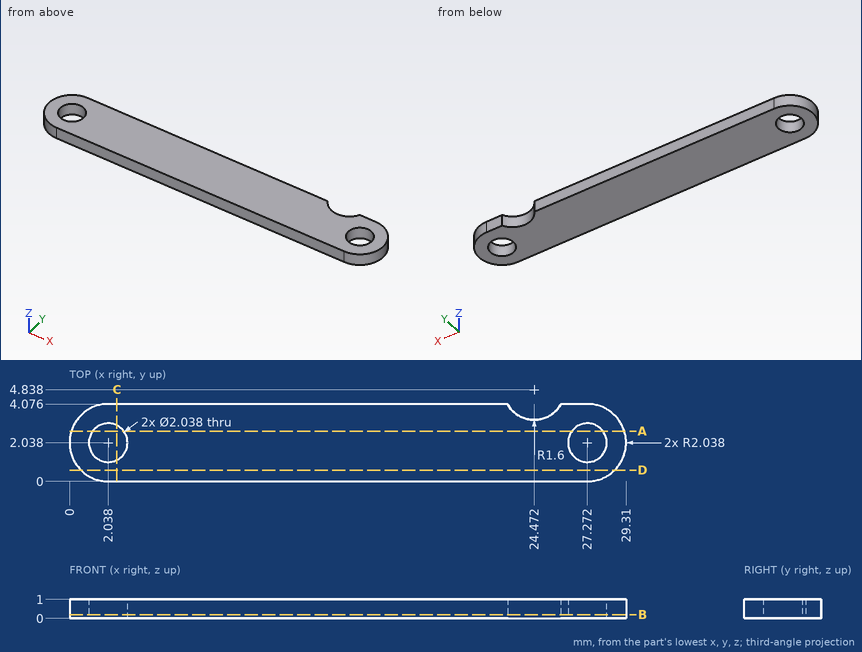
Check sheet for the drawn part. Datum: minimum x, y, z corner. Units: mm. Round coordinates to 2 decimals unless told otherwise and drop trailing zeros. Order: outer loops, then holes, each group sorted by start corner. A loop starts at its lowest first (then second) coordinate and runs counter-clockwise, first axis right, second up. Notation, with made-up numbers: M 20.5,-33.75 L 24.5,-33.75 A21 ccw 24.5,0.25 Z; hole C -32.75,74 d2. An arc over 180 degrees is marked long. Write each question's results on one line, items separated by ' | '. Start each with the question number.
1. Cross-section at D-D on y = 0.6. Record the boundary of the cut face in (x, z).
2. Cross-section at A-A on y = 2.65. Record the boundary of the cut face in (x, z).
3. Cross-section at B-B on z = 0.2. Record the boundary of the cut face in (x, y) (1 decimal).
4. Material ranges on L1, parallel to X at y = 2, z = 0.75; L2, parallel to X at y = 2.7, z = 0.15 (1 decimal); L3, parallel to Y at x = 2.75, z = 0.1 (1 decimal), recorded low to high. Write a range as from..to.
5. Cross-section at C-C on x = 2.5. Record the boundary of the cut face in (y, z).
Resolved:
1) outline: M 0.59,0 L 28.72,0 L 28.72,1 L 0.59,1 Z
2) outline: M 0.09,0 L 1.22,0 L 1.22,1 L 0.09,1 Z; M 2.85,0 L 26.46,0 L 26.46,1 L 2.85,1 Z; M 28.09,0 L 29.22,0 L 29.22,1 L 28.09,1 Z
3) outline: M 2,0 L 27.3,0 A2 ccw 27.3,4.1 L 25.9,4.1 A1.6 cw 23.1,4.1 L 2,4.1 A2 ccw Z; hole C 2,2 d2; hole C 27.3,2 d2
4) L1: 0..1.02, 3.06..26.25, 28.29..29.31 | L2: 0.1..1.3, 2.8..26.5, 28..29.2 | L3: 0..1.3, 2.8..4.1
5) outline: M 0,0 L 1.13,0 L 1.13,1 L 0,1 Z; M 2.95,0 L 4.08,0 L 4.08,1 L 2.95,1 Z
